```python
from build123d import *
from OCP.BRepFilletAPI import BRepFilletAPI_MakeChamfer

# Parameters (mm, degrees)
BOSS_EXTRUDE1_DEPTH = 20
SKETCH2_W           = 641.5
SKETCH2_H           = 23
SKETCH2_W_2         = 611.1
SKETCH2_H_2         = 8.73125
BOSS_EXTRUDE2_DEPTH = 6.35
SKETCH4_W           = 80
SKETCH4_H           = 19.05
BOSS_EXTRUDE3_DEPTH = 40
CUT_EXTRUDE2_DEPTH  = 50.8
CHAMFER1_SIZE       = 20
CHAMFER1_SIZE_2     = 3.526539614
SKETCH2_3_W         = 305.55
SKETCH2_3_H         = 8.73125
CUT_EXTRUDE3_DEPTH  = 20
FILLET1_R           = 10


with BuildPart() as part:
    # Sketch1 → Boss-Extrude1 (new body)
    with BuildSketch(Plane(origin=(0, 0, 0), x_dir=(1, 0, 0), z_dir=(0, 1, 0))):
        Polygon((-341.35, 23), (-341.35, 7.291), (-320.75, 7.291), (-320.75, -7.291), (-341.35, -7.291), (-341.35, -23), (341.35, -23), (341.35, -7.291), (320.75, -7.291), (320.75, 7.291), (341.35, 7.291), (341.35, 23), align=None)
    extrude(amount=BOSS_EXTRUDE1_DEPTH)

    # Sketch2 → Boss-Extrude2 (add)
    with BuildSketch(Plane(origin=(0, 20, 0), x_dir=(1, 0, 0), z_dir=(0, 1, 0))):
        with Locations((0, -11.5)):
            Rectangle(SKETCH2_W, SKETCH2_H)
        with Locations((0, -12.284375)):
            Rectangle(SKETCH2_W_2, SKETCH2_H_2, mode=Mode.SUBTRACT)
    extrude(amount=BOSS_EXTRUDE2_DEPTH)

    # Sketch4 → Boss-Extrude3 (add)
    with BuildSketch(Plane(origin=(0, 20, 0), x_dir=(1, 0, 0), z_dir=(0, 1, 0))):
        with Locations((0, 13.475)):
            Rectangle(SKETCH4_W, SKETCH4_H)
    extrude(amount=BOSS_EXTRUDE3_DEPTH)

    # Sketch5 → Cut-Extrude2 (cut)
    with BuildSketch(Plane(origin=(0, 0, -23), x_dir=(-1, 0, 0), z_dir=(0, 0, -1))):
        with BuildLine():
            ThreePointArc((3.407767598, 41.703883799), (0, 43.81), (-3.407767598, 41.703883799))
            Line((-3.407767598, 41.703883799), (0, 40))
            Line((0, 40), (3.407767598, 41.703883799))
        make_face()
        with BuildLine():
            Line((0, 40), (-3.407767598, 41.703883799))
            ThreePointArc((-3.407767598, 41.703883799), (-3.81, 40), (-3.407767598, 38.296116201))
            Line((-3.407767598, 38.296116201), (0, 40))
        make_face()
        with BuildLine():
            Line((3.407767598, 41.703883799), (0, 40))
            Line((0, 40), (3.407767598, 38.296116201))
            ThreePointArc((3.407767598, 38.296116201), (3.70807865, 39.124641373), (3.81, 40))
            ThreePointArc((3.81, 40), (3.70807865, 40.875358627), (3.407767598, 41.703883799))
        make_face()
        with BuildLine():
            Line((3.407767598, 38.296116201), (0, 40))
            Line((0, 40), (-3.407767598, 38.296116201))
            ThreePointArc((-3.407767598, 38.296116201), (0, 36.19), (3.407767598, 38.296116201))
        make_face()
    extrude(amount=-CUT_EXTRUDE2_DEPTH, mode=Mode.SUBTRACT)

    # Chamfer1
    chamfer1_edges_1 = [part.edges().sort_by_distance(p)[0] for p in [
        (331.05, 0, -7.291),
    ]]
    chamfer1_side_1 = [part.faces().sort_by_distance(p)[0] for p in [
        (331.05, 0.070530792, -7.291),
    ]]
    chamfer1_edges_2 = [part.edges().sort_by_distance(p)[0] for p in [
        (331.05, 0, 7.291),
    ]]
    chamfer1_side_2 = [part.faces().sort_by_distance(p)[0] for p in [
        (331.05, 0, 7.361530792),
    ]]
    chamfer1_edges_3 = [part.edges().sort_by_distance(p)[0] for p in [
        (-331.05, 0, 7.291),
    ]]
    chamfer1_side_3 = [part.faces().sort_by_distance(p)[0] for p in [
        (-331.05, 0, 7.361530792),
    ]]
    chamfer1_edges_4 = [part.edges().sort_by_distance(p)[0] for p in [
        (-331.05, 0, -7.291),
    ]]
    chamfer1_side_4 = [part.faces().sort_by_distance(p)[0] for p in [
        (-331.05, 0, -7.361530792),
    ]]
    chamfer1 = BRepFilletAPI_MakeChamfer(part.part.solid().wrapped)
    for e in chamfer1_edges_1:
        chamfer1.Add(CHAMFER1_SIZE - 0.0001, CHAMFER1_SIZE_2 - 0.0001, e.wrapped, chamfer1_side_1[0].wrapped)
    for e in chamfer1_edges_2:
        chamfer1.Add(CHAMFER1_SIZE_2 - 0.0001, CHAMFER1_SIZE - 0.0001, e.wrapped, chamfer1_side_2[0].wrapped)
    for e in chamfer1_edges_3:
        chamfer1.Add(CHAMFER1_SIZE_2 - 0.0001, CHAMFER1_SIZE - 0.0001, e.wrapped, chamfer1_side_3[0].wrapped)
    for e in chamfer1_edges_4:
        chamfer1.Add(CHAMFER1_SIZE_2 - 0.0001, CHAMFER1_SIZE - 0.0001, e.wrapped, chamfer1_side_4[0].wrapped)
    add(Compound.cast(chamfer1.Shape()), mode=Mode.REPLACE)  # a hair under: the kernel refuses the full size

    # Sketch2<3> → Cut-Extrude3 (cut)
    with BuildSketch(Plane(origin=(0, 20, 0), x_dir=(1, 0, 0), z_dir=(0, 1, 0))):
        with Locations((-152.775, -12.284375)):
            Rectangle(SKETCH2_3_W, SKETCH2_3_H)
        with Locations((152.775, -12.284375)):
            Rectangle(SKETCH2_3_W, SKETCH2_3_H)
    extrude(amount=-CUT_EXTRUDE3_DEPTH, mode=Mode.SUBTRACT)

    # Fillet1
    fillet1_edges = [part.edges().sort_by_distance(p)[0] for p in [
        (40, 20, -13.475),
        (-40, 60, -13.475),
        (40, 60, -13.475),
        (-40, 20, -13.475),
    ]]
    fillet(fillet1_edges, radius=FILLET1_R)


solid = part.part
```
The listing builds one solid part. Answer for the finished solid, in the listing's coordinates (mm). A direction names the side the tool comes from. Coordinates: 2 decimals unless noted, no trailing zeros. Write each loop counter-clockwise with the first axis right and the second up, starting at its lowest first coordinate (ties: lowest second). Pieces come first, ordered by that corner, then holes. Notation, with made-up numbers: (-5.75, -2.5) -> (24.25, -2.5) arc R22 ccw to (24.25, 5.5) -> close; hole circle Ø2 at (53, -23.5). An arc over 180 degrees is marked (long way). Write each question's results on one line, items separated by ' | '. Start each with the question number.
1) A cutting plane is placed at A-A (x = 274). Determine the outline of the cut face in (y, z).
2) A tool of negligible diameter and unlimited length cuts with its end or side. For faces 4 (the flat face through (-40, 40, -13)), 5 (the flat face through (331.19, 10.14, 9.03)), 6 (the flat face through (-4, 13, 16.65)), 7 (the flat face through (-1, 35, -3.95)), from which of +Z, -Z, +X, -X, +Y, -Y can it reach the whole face along a straight path? Write none if from no direction.
3) Flat-ended cylindrical pins translate along their axes: pin 1 Ø4.5 at (x, z) = (330, 18) entering from +Y; pin 2 Ø10 at (y, z) = (31, -17.5) entering from -X; pin 3 Ø11.5 at (x, z) = (126.5, 12) entering from +Y. Find the tip coordinate at first contact, or state that the pin passes through.
4) For a pull along Z with two mould halves and no side action, classify faces 1 (the flat face through (0, 60, -14)), 2 (the flat face through (5, 16, -23)), 3 (the flat face through (-330.91, 10.14, 9.03)) as +Z half, -Z half, draft (parallel to the pull), parting line (faces both ways), or undercut.
5) Straight lines are drawn through the part: probe 1 along Z at (x, y) = (-47, 6); probe 2 along X at (y, z) = (3, 8); probe 3 along Y at (x, z) = (109, 1). For each, find the intervals that lie inside material, in ascending order.
Values follow:
1) outline: (0, -23) -> (20, -23) -> (20, 0) -> (26.35, 0) -> (26.35, 7.92) -> (0, 7.92) -> close; (0, 16.65) -> (26.35, 16.65) -> (26.35, 23) -> (0, 23) -> close
2) face 4: +Z, -Z, -X, +Y | face 5: +X, -Y | face 6: +Y, -Y | face 7: +X, -X, +Y
3) pin 1: y = 20 | pin 2: x = -40.83 | pin 3: y = 26.35
4) face 1: draft | face 2: -Z half | face 3: undercut
5) probe 1: -23 to 7.92, 16.65 to 23 | probe 2: -320.75 to -305.55, 305.55 to 320.75 | probe 3: 0 to 26.35
